The drawing under review shows one solid part. Ordinate dimensions are in mm from its lowest x, y, z. Give positions to 0.01 mm unless a question says otherwise; leave off trailing zeros. Loops run counter-clockwise (first coordinate to the right, second up) from the corner with the lowest first, then second, coordinate; pieces in that order, holes last. Notation, with made-up numbers: (33, 43) -> (44, 43) arc R36 cw to (44, 82) -> close; hole circle Ø6 at (-26.75, -27). An arc over 180 degrees is marked (long way). Answer in a Markdown table with one row per item. Add a question column.
(1) For line 1 (Z direction, x = 2.3, y = 14.25); line 2 (Z direction, x = 1.6, y = 23) (1 decimal); line 3 (Y direction, x = 0.35, z = 26) (1 decimal), list the stretches that pass through material, from the lowest coordinate up.
(2) Consider section A-A on x = 0.85. Write out the cut boundary in (y, z), then the cut area to 3 significant figures.
(3) Draft analysis for pull direction Z (two halves, no side actions). For the marked faces 1, 2 and 3, state which applies: +Z half, -Z half, draft (parallel to the pull), parting line (faces both ways), or undercut.
(4) For pin 1 (1.5 mm diameter, centred on x = 1.5, z = 15, fed in from +Y); pin 2 (1.5 mm diameter, centred on x = 0.5, y = 5.5, fed in from +Z) (1 decimal), all flat-tipped, find the tip position at first contact; note any pin that passes through.
(5) Consider section B-B on y = 10.75. Write out the cut boundary in (x, z).
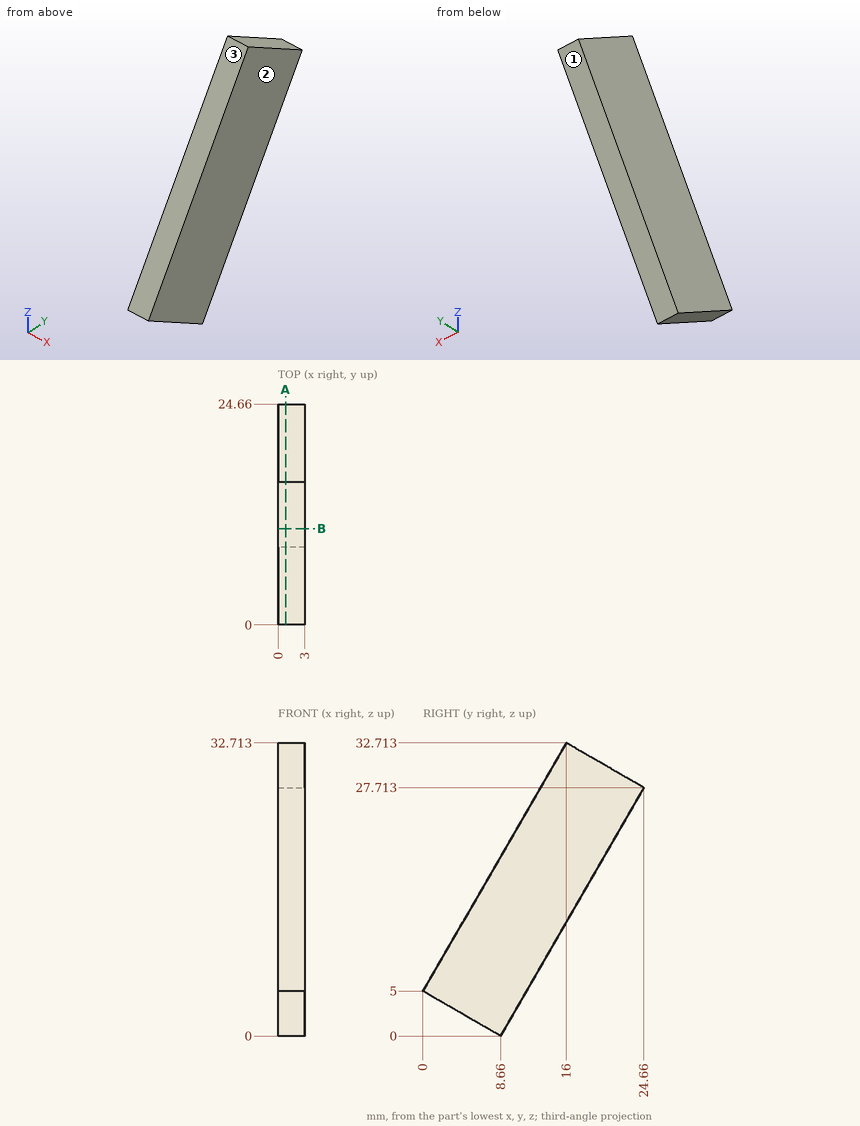
Values follow:
| question | item | result |
|---|---|---|
| 1 | line 1 | 9.68 to 29.68 |
| 1 | line 2 | 24.8 to 28.7 |
| 1 | line 3 | 12.1 to 23.7 |
| 2 | outline | (0, 5) -> (8.66, 0) -> (24.66, 27.71) -> (16, 32.71) -> close |
| 2 | area | 320 mm2 |
| 3 | face 1 | -Z half |
| 3 | face 2 | draft |
| 3 | face 3 | +Z half |
| 4 | pin 1 | y = 17.75 |
| 4 | pin 2 | z = 15.8 |
| 5 | outline | (0, 3.62) -> (3, 3.62) -> (3, 23.62) -> (0, 23.62) -> close |
